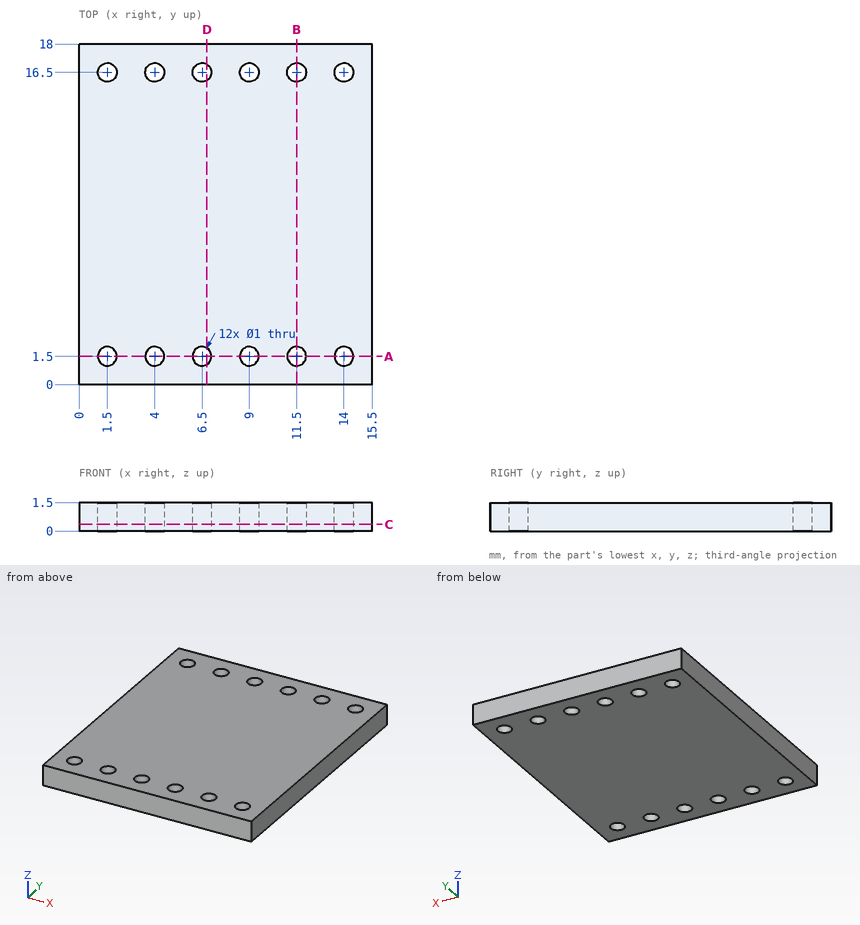
Drawing for the job (mm, zero at the part's lowest x, y, z). Round coordinates to 2 decimals unless told otherwise and drop trailing zeros. Loops run counter-clockwise (first coordinate to the right, second up) from the corner with the lowest first, then second, coordinate; pieces in that order, holes last. Notation, with made-up numbers: (-32.75, -37) -> (-19.75, -37) arc R17 ccw to (-19.75, -9) -> close; hole circle Ø7 at (0.5, 10.5). An arc over 180 degrees is marked (long way). Answer as CSV lines item,"result". Start each with the question number.
1) Slice it at B-B (x = 11.5). List the corners of the cut face in (y, z), plus the area to 3 significant figures.
2) Slice it at D-D (x = 6.75). List the corners of the cut face in (y, z), plus the area to 3 significant figures.
3) Probe line 1 along Y through (x, z) = (1.5, 0.4); line 2 along Y through (x, z) = (13.75, 0.3). List the from-to ranges inside material, lowest first.
4) Slice it at A-A (y = 1.5). List the corners of the cut face in (x, z), plus the area to 4 significant figures.
5) Slice it at C-C (z = 0.35). State how many separate pieces and enclosed holes the cut face has, plus the area to 3 significant figures.
Filled in:
1,outline,"(0, 0) -> (1, 0) -> (1, 1.5) -> (0, 1.5) -> close; (2, 0) -> (16, 0) -> (16, 1.5) -> (2, 1.5) -> close; (17, 0) -> (18, 0) -> (18, 1.5) -> (17, 1.5) -> close"
1,area,"24.0 mm2"
2,outline,"(0, 0) -> (1.07, 0) -> (1.07, 1.5) -> (0, 1.5) -> close; (1.93, 0) -> (16.07, 0) -> (16.07, 1.5) -> (1.93, 1.5) -> close; (16.93, 0) -> (18, 0) -> (18, 1.5) -> (16.93, 1.5) -> close"
2,area,"24.4 mm2"
3,line 1,"y = 0 to 1, 2 to 16, 17 to 18"
3,line 2,"y = 0 to 1.07, 1.93 to 16.07, 16.93 to 18"
4,outline,"(0, 0) -> (1, 0) -> (1, 1.5) -> (0, 1.5) -> close; (2, 0) -> (3.5, 0) -> (3.5, 1.5) -> (2, 1.5) -> close; (4.5, 0) -> (6, 0) -> (6, 1.5) -> (4.5, 1.5) -> close; (7, 0) -> (8.5, 0) -> (8.5, 1.5) -> (7, 1.5) -> close; (9.5, 0) -> (11, 0) -> (11, 1.5) -> (9.5, 1.5) -> close; (12, 0) -> (13.5, 0) -> (13.5, 1.5) -> (12, 1.5) -> close; (14.5, 0) -> (15.5, 0) -> (15.5, 1.5) -> (14.5, 1.5) -> close"
4,area,"14.25 mm2"
5,separate pieces,"1"
5,enclosed holes,"12"
5,area,"270 mm2"
